Work out the finished part from the listing and answer in its coordinate system (mm). Give positions to 0.01 mm unless a question says otherwise; leave off trailing zeros. One line per question, with ' | ' between items. Start each with the question number.
1. Section A-A (x = 11) is taken. Give the number of separate pieces and of enclosed holes in the cut face, plus the area to 3 significant figures.
2. Find the intervals of material crossed by line 1 (Z direction, x = -8, y = -5.5); line 2 (Z direction, x = 5.5, y = -15); line 3 (Y direction, x = 0, z = 6), in increasing order.
3. For a pull along Y with two mould halves and no side action, classify faces 1 (the face through (0, 0, 155)), 2 (the face through (0, 0, 8)), 3 (the face through (-12, 12, 1)) as released by +Y, released by -Y, zero draft, split by the parting line, or undercut.
4. Each of these flat-tipped pins is pushed along its axis until it touches: pin 1 (5 mm diameter, centred on x = 0, y = 0, fed in from +Z); pin 2 (4 mm diameter, centred on x = -9.5, y = 4, fed in from +Z); pin 3 (8 mm diameter, centred on x = 14, z = 33, fed in from +Y); pin 4 (11 mm diameter, centred on x = 0, y = 1.5, fed in from +Z). Where does it stop, or does it pass through?
from build123d import *
from build123d.topology import SkipClean

# Parameters (mm, degrees)
SKETCH_1_R          = 5
EXTRUDE_1_DEPTH     = 155
SWEEP_1_PITCH       = 38.675
SWEEP_1_HEIGHT      = 154.7
SWEEP_1_RADIUS      = 5
SWEEP_1_START_ANGLE = 45
SKETCH_4_W          = 2
SKETCH_4_H          = 24
SKETCH_5_R          = 4
CUT_EXTRUDE_1_DEPTH = 8


with BuildPart() as part:
    # 草图1 → 凸台-拉伸1 (new body)
    with BuildSketch(Plane.XY):
        Circle(SKETCH_1_R)
    extrude(amount=EXTRUDE_1_DEPTH)

    # 扫描1: sweep along a helix
    with SkipClean():  # the faces are left unmerged after this step: merging them gives an invalid solid
        with BuildLine() as sweep_1_path:
            add(Helix(SWEEP_1_PITCH, SWEEP_1_HEIGHT, SWEEP_1_RADIUS, center=(0, 0, 155), direction=(0, 0, -1), mode=Mode.PRIVATE).rotate(Axis((0, 0, 155), (0, 0, -1)), SWEEP_1_START_ANGLE))
        # 草图4 → 扫描1 (sweep)
        with BuildSketch(Plane(origin=(-3.535533906, 3.535533906, 0.3), x_dir=(0, 0, 1), z_dir=(-0.7071067811866223, -0.7071067811864729, 0))):
            with Locations((0.7, 12)):
                Rectangle(SKETCH_4_W, SKETCH_4_H)
        sweep(path=sweep_1_path.line, is_frenet=True)

    # 草图5 → 切除-拉伸1 (cut)
    with SkipClean():  # the faces are left unmerged after this step: merging them gives an invalid solid
        with BuildSketch(Plane(origin=(0, 0, 0), x_dir=(-1, 0, 0), z_dir=(0, 0, -1))):
            Circle(SKETCH_5_R)
        extrude(amount=-CUT_EXTRUDE_1_DEPTH, mode=Mode.SUBTRACT)


solid = part.part
Conclusion:
1) separate pieces: 4 | enclosed holes: 0 | area: 429 mm²
2) line 1: 8.54 to 10.54, 47.22 to 49.22, 85.89 to 87.89, 124.57 to 126.57 | line 2: 16.67 to 18.67, 55.34 to 57.34, 94.02 to 96.02, 132.69 to 134.69 | line 3: -5 to -4, 4 to 5
3) face 1: zero draft | face 2: undercut | face 3: released by +Y
4) pin 1: z = 155 | pin 2: z = 121.61 | pin 3: y = 27.22 | pin 4: z = 156.7
